from build123d import *

# Parameters (mm, degrees)
SKETCH1_R               = 3.4925
BOSS_EXTRUDE1_DEPTH     = 63.5
SKETCH2_W               = 50.8
SKETCH2_H               = 34.925
CUT_EXTRUDE1_DEPTH      = 10.525
CUT_EXTRUDE1_DEPTH_BACK = 60.869090512
BOSS_EXTRUDE2_DEPTH     = 12.7
FILLET2_R               = 40.64


with BuildPart() as part:
    # Sketch1 → Boss-Extrude1 (new body)
    with BuildSketch(Plane.XY):
        with BuildLine():
            Line((-59.869090512, -25.4), (-4.964236422, 8.129082467))
            ThreePointArc((-4.964236422, 8.129082467), (8.292412041, 4.686312788), (4.403021401, -8.446243398))
            Line((4.403021401, -8.446243398), (-28.119090512, -25.4))
            Line((-28.119090512, -25.4), (-28.119090512, -38.1))
            Line((-28.119090512, -38.1), (-59.869090512, -38.1))
            Line((-59.869090512, -38.1), (-59.869090512, -25.4))
        make_face()
        Circle(SKETCH1_R, mode=Mode.SUBTRACT)
    extrude(amount=BOSS_EXTRUDE1_DEPTH)

    # Sketch2 → Cut-Extrude1 (cut, two sides)
    with BuildSketch(Plane(origin=(0, 0, 0), x_dir=(0, 0, -1), z_dir=(1, 0, 0))) as cut_extrude1_sk:
        with Locations((-31.75, -7.9375)):
            Rectangle(SKETCH2_W, SKETCH2_H)
    extrude(amount=CUT_EXTRUDE1_DEPTH, mode=Mode.SUBTRACT)
    extrude(cut_extrude1_sk.sketch, amount=-CUT_EXTRUDE1_DEPTH_BACK, mode=Mode.SUBTRACT)

    # Sketch3 → Boss-Extrude2 (add)
    with BuildSketch(Plane.XZ.offset(38.1)):
        with BuildLine():
            Line((-55.074857205, 63.5), (-59.869090512, 63.5))
            Line((-59.869090512, 63.5), (-59.869090512, 0))
            Line((-59.869090512, 0), (-55.074857205, 0))
            ThreePointArc((-55.074857205, 0), (-41.454090512, 31.75), (-55.074857205, 63.5))
        make_face()
        with BuildLine():
            Line((-44.803095838, 63.5), (-28.119090512, 63.5))
            Line((-28.119090512, 63.5), (-28.119090512, 0))
            Line((-28.119090512, 0), (-44.803095838, 0))
            ThreePointArc((-44.803095838, 0), (-33.834090512, 31.75), (-44.803095838, 63.5))
        make_face()
    extrude(amount=BOSS_EXTRUDE2_DEPTH)

    # Fillet2
    fillet2_edges = [part.edges().sort_by_distance(p)[0] for p in [
        (-28.119090512, -25.4, 60.325),
        (-28.119090512, -25.4, 3.175),
    ]]
    fillet(fillet2_edges, radius=FILLET2_R)


solid = part.part
Model file for the job. Use its own axes, mm. A direction names the side the tool comes from. Give positions to 0.01 mm unless a question says otherwise; leave off trailing zeros. Write each loop counter-clockwise with the first axis right and the second up, starting at its lowest first coordinate (ties: lowest second). Pieces come first, ordered by that corner, then holes. Notation, with made-up numbers: (-31, -36) -> (-1, -36) arc R24 ccw to (-1, -16) -> close; hole circle Ø11 at (66.5, -21.5). An arc over 180 degrees is marked (long way). Write item = value, one per line.
(1) Slice it at C-C, the plane y = 0. Give the number of separate pieces and of enclosed holes in the cut face, then the cut area to 3 significant figures.
Determined:
separate_pieces = 4
enclosed_holes = 0
area = 264 mm2
(2) Probe line 1 along Z through (x, y) = (5, 7.5); line 2 along Y through (x, z) = (-54, 44.5); line 3 along Y through (x, z) = (-41.5, 9). List the from-to ranges inside material, lowest first.
Determined:
line_1 = 0 to 6.35, 57.15 to 63.5
line_2 = -50.8 to -25.4
line_3 = -38.1 to -25.4
(3) Tool access for faces 1 (the face through (-40, -38.1, 31)), 2 (the face through (-32.8, -8.87, 3.13)): list every direction of +Z, -Z, +X, -X, +Y, -Y with a clear straight run to the whole face (end or side of a thin tool).
Determined:
face_1 = -Y
face_2 = +Z, -Z, -X, +Y
(4) Mould opens along X. For faces 3 (the face through (-0.455, 3.463, 3.131)), 4 (the face through (-28.119, -38, 31)), 5 (the face through (-32.8, -8.87, 60.28)), 6 (the face through (-26, -20, 0)) say: released by +X, released by -X, zero draft, split by the parting line, or undercut.
Determined:
face_3 = undercut
face_4 = released by +X
face_5 = released by -X
face_6 = zero draft
(5) Slice it at B-B, the plane x = -17. Give the cut face in (y, z), then the cut area to 3 significant figures.
Determined:
outline = (-22.11, 0) -> (0.78, 0) -> (0.78, 6.35) -> (-22.11, 6.35) -> close; (-22.11, 57.15) -> (0.78, 57.15) -> (0.78, 63.5) -> (-22.11, 63.5) -> close
area = 291 mm2
(6) Flat gauge pins, fed straight in: P1, Ø16, axis at x = -51, z = 31.5, coming from the +Y side; P2, Ø20.5, axis at y = -37, z = 30.5, coming from the +X side. Where does each tip first touch, or does it go through?
Determined:
P1 = -25.4
P2 = -28.12
(7) Slice it at A-A, the plane y = -10.5. Give the cut face in (x, z).
Determined:
outline = (-35.47, 0) -> (0.46, 0) -> (0.46, 6.35) -> (-35.47, 6.35) -> close; (-35.47, 57.15) -> (0.46, 57.15) -> (0.46, 63.5) -> (-35.47, 63.5) -> close
